Autodesk Inventor part; units mm, degrees
ref_plane "YZ Plane" through (0, 0, 0) normal (1, 0, 0) x (0, 1, 0)
ref_plane "XZ Plane" through (0, 0, 0) normal (0, 1, 0) x (-1, 0, 0)
ref_plane "XY Plane" through (0, 0, 0) normal (0, 0, 1) x (1, 0, 0)
sketch "Skizze1" plane through (0, 0, 0) normal (0, 0, 1) x (1, 0, 0)
  line L0 (-11.2, 0) -> (11.2, 0)
  line L1 (0, -11.2) -> (0, 11.2)
  circle A0 centre (0, 0) radius 8
  circle A1 centre (0, 0) radius 2.5
  dimension "d0" = 16
  dimension "d1" = 5
extrude "Extrusion1" add sketch "Skizze1" along normal mid plane 5 contours A1 L1 A0 L0 | L0 A0 L1 A1 | A1 L0 A0 L1 | L1 A0 L0 A1
sketch "Skizze2" plane through (0, 0, 2.5) normal (0, 0, 1) x (1, 0, 0)
  circle A0 centre (0, 0) radius 2.5
  circle A1 centre (0, 0) radius 8
  circle A2 centre (0, 0) radius 3.5
  circle A3 centre (0, 0) radius 7
  dimension "d4" = 7
  dimension "d5" = 14
extrude "Extrusion2" cut sketch "Skizze2" against normal blind 0.2 contours A3
mirror "Spiegeln1" about plane through (0, 0, 0) normal (0, 0, 1) of "Extrusion2"
chamfer "Fase1" distance 0.05 angle 45 1 edges at (-7, 0, 2.5)
chamfer "Fase2" distance 0.05 angle 45 1 edges at (-3.5, 0, 2.5)
chamfer "Fase3" distance 0.05 angle 45 1 edges at (-2.5, 0, 2.5)
chamfer "Fase4" distance 0.05 angle 45 1 edges at (-8, 0, 2.5)
chamfer "Fase5" distance 0.05 angle 45 1 edges at (-8, 0, -2.5)
chamfer "Fase6" distance 0.05 angle 45 1 edges at (-7, 0, -2.5)
chamfer "Fase7" distance 0.05 angle 45 1 edges at (-3.5, 0, -2.5)
chamfer "Fase8" distance 0.05 angle 45 1 edges at (-2.5, 0, -2.5)
properties part number "Kugellager625_5x16x5" material "Stahl, Kohlenstoff"
The listing builds one solid part. Answer for the finished solid, in the listing's coordinates (mm). Give positions to 0.01 mm unless a question says otherwise; leave off trailing zeros. Write each loop counter-clockwise with the first axis right and the second up, starting at its lowest first coordinate (ties: lowest second). Pieces come first, ordered by that corner, then holes.
Item 1: Section A-A, the plane z = -0.75 is taken. Write down the section's boundary in (x, y).
Item 2: Flat-ended cylindrical pins translate along their axes: P1, Ø3, axis at x = 0, y = 0, coming from the +Z side; P2, Ø1.5, axis at x = 3.5, y = 4, coming from the -Z side; P3, Ø3, axis at y = 3.5, z = 1, coming from the +X side. Find the tip coordinate at first contact, or state that the pin passes through.
Item 3: Determine the mould class of faces 1 (the flat face through (3, -3, 2.3)), 2 (the cylindrical face through (-1.73, -7.81, 0.03)), 3 (the cylindrical face through (-0.54, 2.44, -0.03)), 4 (the flat face through (0, -3, 2.5)) for opening direction Y: released by +Y, released by -Y, zero draft, split by the parting line, or undercut.
Item 4: Find the intervals of material crossed by line 1 along Y through (x, z) = (0, -2.35); line 2 along X through (y, z) = (0, 1.05); line 3 along Z through (x, y) = (6.25, -2), in increasing order.
Completed:
1. outline: circle Ø16 at (0, 0); hole circle Ø5 at (0, 0)
2. P1: passes through
2. P2: stops at z = -2.3
2. P3: stops at x = 7.75
3. face 1: undercut
3. face 2: split by the parting line
3. face 3: undercut
3. face 4: zero draft
4. line 1: y = -8 to -7, -3.5 to -2.5, 2.5 to 3.5, 7 to 8
4. line 2: x = -8 to -2.5, 2.5 to 8
4. line 3: z = -2.3 to 2.3
